```python
from build123d import *

# Parameters (mm, degrees)
BOSS_EXTRUDE1_DEPTH = 3.175


with BuildPart() as part:
    # Sketch1 → Boss-Extrude1 (new body)
    with BuildSketch(Plane.XY):
        Polygon((257.81, 76.2), (222.25, 76.2), (222.25, 0), (0, 0), (0, 101.6), (63.5, 101.6), (63.5, 19.05), (165.1, 19.05), (165.1, 101.6), (257.81, 101.6), align=None)
    extrude(amount=BOSS_EXTRUDE1_DEPTH)


solid = part.part
```
Input: part model. Units: mm. Frame: model coordinates. Coordinates: 2 decimals unless noted, no trailing zeros. Write each loop counter-clockwise with the first axis right and the second up, starting at its lowest first coordinate (ties: lowest second). Pieces come first, ordered by that corner, then holes. Notation, with made-up numbers: (-11, 20.25) -> (38, 20.25) arc R24 ccw to (38, 50.25) -> close; hole circle Ø9 at (35.5, 53.5). An arc over 180 degrees is marked (long way). Answer as a JSON object with one key per item and string values.
1. First-contact query: P1, Ø1.5, axis at x = 158, z = 2.5, coming from the +Y side; P2, Ø1.6, axis at x = 244.5, z = 1.5, coming from the -Y side; P3, Ø1, axis at y = 64.5, z = 1.5, coming from the +X side. Flat tips, straight axial feed; report the tip coordinate or a pass-through.
Result set:
{"P1": "stops at y = 19.05", "P2": "stops at y = 76.2", "P3": "stops at x = 222.25"}
2. Section B-B on z = 2.2. Return the cut outline in (x, y), then the cut area to 3 significant figures.
Result set:
{"outline": "(0, 0) -> (222.25, 0) -> (222.25, 76.2) -> (257.81, 76.2) -> (257.81, 101.6) -> (165.1, 101.6) -> (165.1, 19.05) -> (63.5, 19.05) -> (63.5, 101.6) -> (0, 101.6) -> close", "area": "15,100 mm2"}
3. Section D-D on x = 92. Return the cut outline in (y, z) (3 decimals), then the cut area to 3 significant figures.
Result set:
{"outline": "(0, 0) -> (19.05, 0) -> (19.05, 3.175) -> (0, 3.175) -> close", "area": "60.5 mm2"}
4. Section C-C on y = 84. Return the cut outline in (x, z) (3 decimals), then the cut area to 3 significant figures.
Result set:
{"outline": "(0, 0) -> (63.5, 0) -> (63.5, 3.175) -> (0, 3.175) -> close; (165.1, 0) -> (257.81, 0) -> (257.81, 3.175) -> (165.1, 3.175) -> close", "area": "496 mm2"}
5. Material intervals for line 1 (X direction, y = 81, z = 2.8); line 2 (X direction, y = 32.5, z = 1.5); line 3 (Y direction, x = 64.5, z = 1.7), sorted ascending. Write a range as from..to.
Result set:
{"line 1": "x = 0..63.5, 165.1..257.81", "line 2": "x = 0..63.5, 165.1..222.25", "line 3": "y = 0..19.05"}
6. Section A-A on y = 51.5. Return the cut outline in (x, z) (3 decimals).
Result set:
{"outline": "(0, 0) -> (63.5, 0) -> (63.5, 3.175) -> (0, 3.175) -> close; (165.1, 0) -> (222.25, 0) -> (222.25, 3.175) -> (165.1, 3.175) -> close"}
